Source: CAD feature listing. Evaluate the final solid. Frame: model axes, mm. Face numbers are marked on the shaded views. A direction names the side the tool comes from. Give positions to 0.01 mm unless a question says otherwise; leave off trailing zeros. Loops run counter-clockwise (first coordinate to the right, second up) from the corner with the lowest first, then second, coordinate; pieces in that order, holes last. Notation, with made-up numbers: M 83,-6.5 L 88,-6.5 A28 ccw 88,20.5 Z; hole C 67,27 d3. An arc over 180 degrees is marked long. Put each result on its own line as item: value.
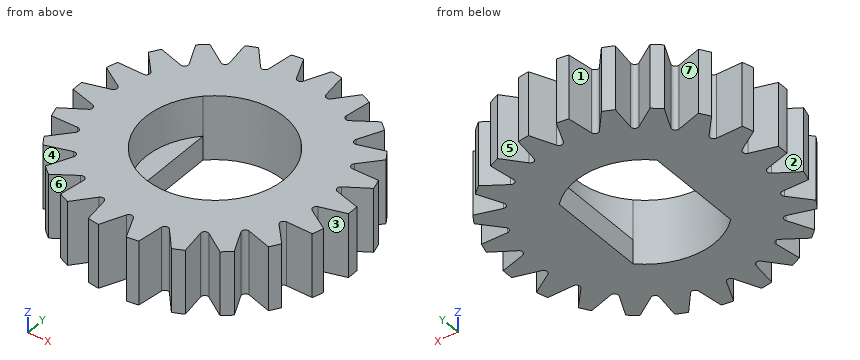
from build123d import *

# Parameters (mm, degrees)
F0_R            = 10.909800859
F1_DEPTH        = 5.08
F3_DEPTH        = 5.08
F3_COPIES_COUNT = 22
F4_R            = 5.5
F5_DEPTH        = 3.175


# Not quite as in the source:
# - a pattern or mirror of a feature is missing from the dataset's text; its kind, count and spacing are read off the source's solid


with BuildPart() as f1:
    # F0 (on Top) → F1 (new body)
    with BuildSketch(Plane.XY):
        Circle(F0_R)
        with BuildLine():
            ThreePointArc((3.8749986, -3.9031251389), (0, -5.5), (-3.8749986, -3.9031251389))
            Line((-3.8749986, -3.9031251389), (-3.8749986, 3.9031251389))
            ThreePointArc((-3.8749986, 3.9031251389), (0, 5.5), (3.8749986, 3.9031251389))
            Line((3.8749986, 3.9031251389), (3.8749986, -3.9031251389))
        make_face(mode=Mode.SUBTRACT)
    extrude(amount=F1_DEPTH)

    # F2 (on face) → F3 (cut, through all)
    with BuildSketch(Plane.XY.offset(5.08)):
        with BuildLine():
            Line((0.2718847261, 8.9821943232), (1.1039126824, 10.8538072386))
            ThreePointArc((1.1039126824, 10.8538072386), (0, 10.909800859), (-1.1039126824, 10.8538072386))
            Line((-1.1039126824, 10.8538072386), (-0.2718847261, 8.9821943232))
            ThreePointArc((-0.2718847261, 8.9821943232), (0, 8.8055210085), (0.2718847261, 8.9821943232))
        make_face()
    f3 = extrude(amount=-F3_DEPTH, mode=Mode.SUBTRACT)

    # F3_copies: F3 ×22 about axis
    f3_copies_axis = Axis((0, 0, 0), (0, 0, 1))
    for i in range(1, F3_COPIES_COUNT):
        add(f3.rotate(f3_copies_axis, i * 360 / F3_COPIES_COUNT), mode=Mode.SUBTRACT)

    # F4 (on face) → F5 (cut)
    with BuildSketch(Plane.XY.offset(5.08)):
        Circle(F4_R)
    extrude(amount=-F5_DEPTH, mode=Mode.SUBTRACT)


solid = f1.part
1. Contact query for flat-ended pins moving along their axis: P1, Ø3, axis at x = -5, z = 3.5, coming from the -Y side; P2, Ø1.5, axis at y = 1, z = 1, coming from the +X side; P3, Ø1.5, axis at x = 7.5, z = 4.5, coming from the +Y side. Output: stop coordinate, or through.
Found:
P1: y = -10.1
P2: x = 10.91
P3: y = 8.53
2. Material intervals for line 1 (Y direction, x = -7, z = 3.15); line 2 (X direction, y = -3.75, z = 0.75) (3 decimals); line 3 (Y direction, x = 9.5, z = 0.8), sorted ascending. Write a range as from..to.
Found:
line 1: -8.37..-6.92, -5.69..5.69, 6.92..8.37
line 2: -7.985..-3.875, 3.875..7.985
line 3: -3.5..-1.95, -0.85..0.85, 1.95..3.5
3. Section query A-A (y = -5.25). Output: boundary loops of the cut face in (x, z), plus the area to 3 significant figures.
Found:
outline: M -9.18,0 L -1.64,0 L -1.64,5.08 L -9.18,5.08 Z; M 1.64,0 L 9.18,0 L 9.18,5.08 L 1.64,5.08 Z
area: 76.6 mm^2
4. Access query for the marked faces 1, 2, 3 and 4. Directions: +Z, -Z, +X, -X, +Y, -Y. A direction counts if a zero-diameter tool reaches every point of the face in a straight line with its end or side. Return the directions, or none.
Found:
face 1: +Z, -Z, +Y
face 2: +Z, -Z, -X
face 3: +Z, -Z, +X
face 4: +Z, -Z
5. Draft query along Y for the marked faces 5, 6 and 7. Return one class per face: pulls with the +Y half, pulls with the -Y half, needs draft (parallel to the pull), parting line crosses it, or undercut.
Found:
face 5: pulls with the +Y half
face 6: pulls with the -Y half
face 7: undercut
